Model file for the job. Use its own axes, mm. Face numbers are marked on the shaded views. A direction names the side the tool comes from. Coordinates: 2 decimals unless noted, no trailing zeros. Order: outer loops, then holes, each group sorted by start corner. A loop starts at its lowest first (then second) coordinate and runs counter-clockwise, first axis right, second up. Notation, with made-up numbers: (32.5, -1) -> (77.5, -1) arc R25 cw to (77.5, 26) -> close; hole circle Ø10 at (13, 57.5). An arc over 180 degrees is marked (long way). Use CSV: the item, a comma, the result in double quotes. Start each with the question number.
(1) Cut at A-A on x = -27.5. Write the cut outline in (y, z), plus the area to 3 significant figures.
(2) Cut at B-B on y = -40. Write the cut outline in (x, z).
(3) Probe L1, parallel to X at y = 32.5, z = -1; L2, parallel to Y at x = -13, z = -2; L3, parallel to X at y = -35.5, z = -0.25. List the from-to ranges inside material, lowest first.
(4) Tool access for the marked faces 1, 2 and 3: list every direction of +Z, -Z, +X, -X, +Y, -Y with a clear straight run to the whole face (end or side of a thin tool).
(5) Pull direction Y, two halves, no side cores. Call the marked faces 4, 5 and 6: pulls with the +Y half, pulls with the -Y half, needs draft (parallel to the pull), parting line crosses it, or undercut.
(6) Cut at C-C on y = -20.5. Write the cut outline in (x, z).
(7) Pin check, flat tips, straight feed: pin 1 Ø1.3 at (x, z) = (-45.5, -1.5) entering from -Y; pin 2 Ø2 at (x, z) = (-11.5, -6) entering from +Y; pin 3 Ø2 at (y, z) = (-45.5, -1.5) entering from -X; pin 4 Ø4.5 at (x, z) = (-47, -1.5) entering from +Y. Stop position of each tip, or through.
```python
from build123d import *

# Parameters (mm, degrees)
F1_DEPTH = 50.8
F3_DEPTH = 7.621
F4_W     = 10.16
F4_H     = 4.064
F5_DEPTH = 12.7
F6_R     = 1.27
F7_DEPTH = 6.35
F8_R     = 0.635
F9_DEPTH = 6.35


# Not quite as in the source:
# - a pattern or mirror of a feature is missing from the dataset's text; its kind, count and spacing are read off the source's solid


with BuildPart() as f1:
    # F0 (on Front) → F1 (new body, symmetric)
    with BuildSketch(Plane.XZ):
        Polygon((-2.54, -4.9092677324), (-2.54, 0.1707322676), (-50.8, 0.1707322676), (-50.8, -4.9092677324), (-45.72, -7.4492677324), align=None)
    extrude(amount=F1_DEPTH, both=True)

    # F2 (on face) → F3 (cut, through all)
    with BuildSketch(Plane.XY.offset(0.1707322676)):
        Polygon((-2.54, 0), (-2.54, 38.1), (-33.02, 38.1), (-33.02, 0), (-33.02, -38.1), (-2.54, -38.1), align=None)
    extrude(amount=-F3_DEPTH, mode=Mode.SUBTRACT)

    # F4 (on face) → F5 (cut)
    with BuildSketch(Plane.XZ.offset(50.8)):
        with Locations((-45.72, -1.8612677324)):
            Rectangle(F4_W, F4_H)
    f5 = extrude(amount=-F5_DEPTH, mode=Mode.SUBTRACT)

    # F5_copies: F5 across plane
    add(f5.mirror(Plane.ZX), mode=Mode.SUBTRACT)

    # F6 (on face) → F7 (join)
    with BuildSketch(Plane.XZ.offset(38.1)):
        with Locations((-45.72, -1.8612677324)):
            Circle(F6_R)
    f7 = extrude(amount=F7_DEPTH)

    # F7_copies: F7 across plane
    add(f7.mirror(Plane.ZX))

    # F8 (on face) → F9 (join)
    with BuildSketch(Plane.XZ.offset(-38.1)):
        with Locations((-19.05, -1.0992677324)):
            Circle(F8_R)
        with Locations((-11.43, -1.0992677324)):
            Circle(F8_R)
    f9 = extrude(amount=F9_DEPTH)

    # F9_copies: F9 across plane
    add(f9.mirror(Plane(origin=(0, 0, 0), x_dir=(0, 0, -1), z_dir=(0, -1, 0))))


solid = f1.part
```
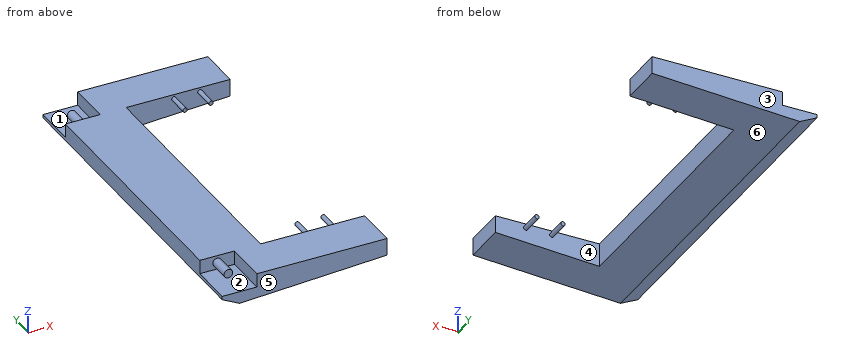
Outcome:
1,outline,"(-50.8, -6.38) -> (-38.1, -6.38) -> (-38.1, 0.17) -> (-50.8, 0.17) -> close; (38.1, -6.38) -> (50.8, -6.38) -> (50.8, 0.17) -> (38.1, 0.17) -> close"
1,area,"166 mm2"
2,outline,"(-50.8, -4.91) -> (-45.72, -7.45) -> (-2.54, -4.91) -> (-2.54, 0.17) -> (-40.64, 0.17) -> (-40.64, -3.89) -> (-50.8, -3.89) -> close; circle Ø2.54 at (-45.72, -1.86)"
3,L1,"-50.8 to -33.02, -19.68 to -18.42, -12.06 to -10.8"
3,L2,"-50.8 to -38.1, 38.1 to 50.8"
3,L3,"-50.8 to -33.02"
4,face 1,"-X, +Y"
4,face 2,"-X, -Y"
4,face 3,"+Z, -Z, +X, -X, +Y"
5,face 4,"undercut"
5,face 5,"pulls with the -Y half"
5,face 6,"needs draft"
6,outline,"(-50.8, -4.91) -> (-45.72, -7.45) -> (-33.02, -6.7) -> (-33.02, 0.17) -> (-50.8, 0.17) -> close"
7,pin 1,"y = -44.45"
7,pin 2,"y = 50.8"
7,pin 3,"x = -40.64"
7,pin 4,"y = 44.45"
